```python
from build123d import *

# Parameters (mm, degrees)
SKETCH_1_R          = 26
EXTRUDE_1_DEPTH     = 7
EXTRUDE_3_DEPTH     = 5
SKETCH_4_R          = 30
SKETCH_4_R_2        = 24
EXTRUDE_4_DEPTH     = 2
EXTRUDE_5_DEPTH     = 7
EXTRUDE_6_DEPTH     = 2
CUT_EXTRUDE_2_DEPTH = 2
SKETCH_11_R         = 1.7
CUT_EXTRUDE_3_DEPTH = 10


with BuildPart() as part:
    # 草图1 → 凸台-拉伸1 (new body)
    with BuildSketch(Plane.XY):
        with BuildLine():
            Line((-15.5, -38), (15.5, -38))
            Line((15.5, -38), (15.5, -25.685599078))
            ThreePointArc((15.5, -25.685599078), (0, 30), (-15.5, -25.685599078))
            Line((-15.5, -25.685599078), (-15.5, -38))
        make_face()
        Circle(SKETCH_1_R, mode=Mode.SUBTRACT)
    extrude(amount=EXTRUDE_1_DEPTH)

    # 草图3 → 凸台-拉伸3 (add)
    with BuildSketch(Plane.XZ.offset(38)):
        with BuildLine():
            Line((-36.263833223, 0), (36.263833223, 0))
            ThreePointArc((36.263833223, 0), (0, 23.12), (-36.263833223, 0))
        make_face()
    extrude(amount=-EXTRUDE_3_DEPTH)

    # 草图4 → 凸台-拉伸4 (add)
    with BuildSketch(Plane.XY.offset(7)):
        Circle(SKETCH_4_R)
        Circle(SKETCH_4_R_2, mode=Mode.SUBTRACT)
    extrude(amount=EXTRUDE_4_DEPTH)

    # 草图5 → 凸台-拉伸5 (add)
    with BuildSketch(Plane(origin=(0, 0, 0), x_dir=(-1, 0, 0), z_dir=(0, 0, -1))):
        with BuildLine():
            Line((-30, -33), (-15.5, -33))
            Line((-15.5, -33), (-15.5, -25.685599078))
            ThreePointArc((-15.5, -25.685599078), (-26.124700955, -14.747881204), (-30, 0))
            Line((-30, 0), (-30, -33))
        make_face()
        with BuildLine():
            Line((15.5, -33), (15.5, -25.685599078))
            ThreePointArc((15.5, -25.685599078), (26.124700955, -14.747881204), (30, 0))
            Line((30, 0), (30, -33))
            Line((30, -33), (15.5, -33))
        make_face()
    extrude(amount=-EXTRUDE_5_DEPTH)

    # 草图8 → 凸台-拉伸6 (add)
    with BuildSketch(Plane.XZ.offset(38)):
        with BuildLine():
            Line((-36.263833223, 0), (36.263833223, 0))
            ThreePointArc((36.263833223, 0), (0, 23.12), (-36.263833223, 0))
        make_face()
    extrude(amount=EXTRUDE_6_DEPTH)

    # 草图9 → 切除-拉伸2 (cut)
    with BuildSketch(Plane(origin=(0, -33, 0), x_dir=(1, 0, 0), z_dir=(0, 1, 0))):
        with BuildLine():
            Line((30, -7), (-30, -7))
            Line((-30, -7), (-30, 0))
            Line((-30, 0), (-36.263833223, 0))
            ThreePointArc((-36.263833223, 0), (0, -23.12), (36.263833223, 0))
            Line((36.263833223, 0), (30, 0))
            Line((30, 0), (30, -7))
        make_face()
    extrude(amount=-CUT_EXTRUDE_2_DEPTH, mode=Mode.SUBTRACT)

    # 草图11 → 切除-拉伸3 (cut)
    with BuildSketch(Plane(origin=(0, -35, 0), x_dir=(1, 0, 0), z_dir=(0, 1, 0))):
        with Locations((-10, -11.85)):
            Circle(SKETCH_11_R)
        with Locations((10, -11.85)):
            Circle(SKETCH_11_R)
    extrude(amount=-CUT_EXTRUDE_3_DEPTH, mode=Mode.SUBTRACT)


solid = part.part
```
Geometry: final body of the model. Coordinates: model frame, mm. A direction names the side the tool comes from. Round coordinates to 2 decimals unless told otherwise and drop trailing zeros. Loops run counter-clockwise (first coordinate to the right, second up) from the corner with the lowest first, then second, coordinate; pieces in that order, holes last.
Item 1: Line query: L1, parallel to X at y = -36.2, z = 11.85; L2, parallel to Y at x = -8, z = 8.25; L3, parallel to Y at x = 0, z = 4.25. Output: solid intervals per line, ascending.
Checked values:
L1: x = -27.83 to -11.7, -8.3 to 8.3, 11.7 to 27.83
L2: y = -40 to -35, -28.91 to -22.63, 22.63 to 28.91
L3: y = -40 to -26, 26 to 30
Item 2: Section D-D, the plane x = -10. Output: boundary loops of the cut face in (y, z).
Checked values:
outline: (-40, 0) - (-24, 0) - (-24, 7) - (-21.82, 7) - (-21.82, 9) - (-28.28, 9) - (-28.28, 7) - (-35, 7) - (-35, 10.15) - (-40, 10.15) - close; (-40, 13.55) - (-35, 13.55) - (-35, 21.85) - (-40, 21.85) - close; (21.82, 7) - (24, 7) - (24, 0) - (28.28, 0) - (28.28, 9) - (21.82, 9) - close
Item 3: Contact query for flat-ended pins moving along their axis: P1, Ø2, axis at y = -15, z = 4, coming from the +X side; P2, Ø2, axis at x = 14, z = 15.5, coming from the +Y side; P3, Ø3.5, axis at y = -20, z = 5, coming from the -X side. Output: stop coordinate, or through.
Checked values:
P1: stops at x = 30
P2: stops at y = -35
P3: stops at x = -30
Item 4: Section A-A, the plane x = 0. Output: boundary loops of the cut face in (y, z).
Checked values:
outline: (-40, 0) - (-26, 0) - (-26, 7) - (-24, 7) - (-24, 9) - (-30, 9) - (-30, 7) - (-35, 7) - (-35, 23.12) - (-40, 23.12) - close; (24, 7) - (26, 7) - (26, 0) - (30, 0) - (30, 9) - (24, 9) - close
Item 5: Section B-B, the plane z = 11.85. Output: boundary loops of the cut face in (x, y), plus the area to 3 significant figures.
Checked values:
outline: (-27.83, -40) - (-11.7, -40) - (-11.7, -35) - (-27.83, -35) - close; (-8.3, -40) - (8.3, -40) - (8.3, -35) - (-8.3, -35) - close; (11.7, -40) - (27.83, -40) - (27.83, -35) - (11.7, -35) - close
area: 244 mm2
Item 6: Mould query, pull axis Y, two halves, no side actions, for faces 1 (the flat face through (0.1, -30.4, 7)), 2 (the flat face through (-1, -40, 9)), 3 (the cylindrical face through (-20.633, -15.821, 3.451)), 4 (the cylindrical face through (-9.086, -37.465, 10.417)). Classes: released by +Y, released by -Y, zero draft, split by the parting line, or undercut.
Checked values:
face 1: undercut
face 2: released by -Y
face 3: undercut
face 4: zero draft
Item 7: Section C-C, the plane y = -20.5. Output: boundary loops of the cut face in (x, z).
Checked values:
outline: (-30, 0) - (-15.99, 0) - (-15.99, 7) - (-12.48, 7) - (-12.48, 9) - (-21.9, 9) - (-21.9, 7) - (-30, 7) - close; (12.48, 7) - (15.99, 7) - (15.99, 0) - (30, 0) - (30, 7) - (21.9, 7) - (21.9, 9) - (12.48, 9) - close
Item 8: Reachability of faces 5 (the flat face through (30, -17, 3)), 6 (the flat face through (-30, -17, 4)), 7 (the flat face through (-13.5, 20.1, 9)), 8 (the flat face through (8, -23, 7)), 9 (the cylindrical face through (-3.905, 29.745, 5.437)) from +Z, -Z, +X, -X, +Y, -Y: full face, straight path, thin tool, end or side. Return the list, or none.
Checked values:
face 5: +Z, -Z, +X, +Y
face 6: +Z, -Z, -X, +Y
face 7: +Z, +X, -X, +Y
face 8: -Z
face 9: +Z
